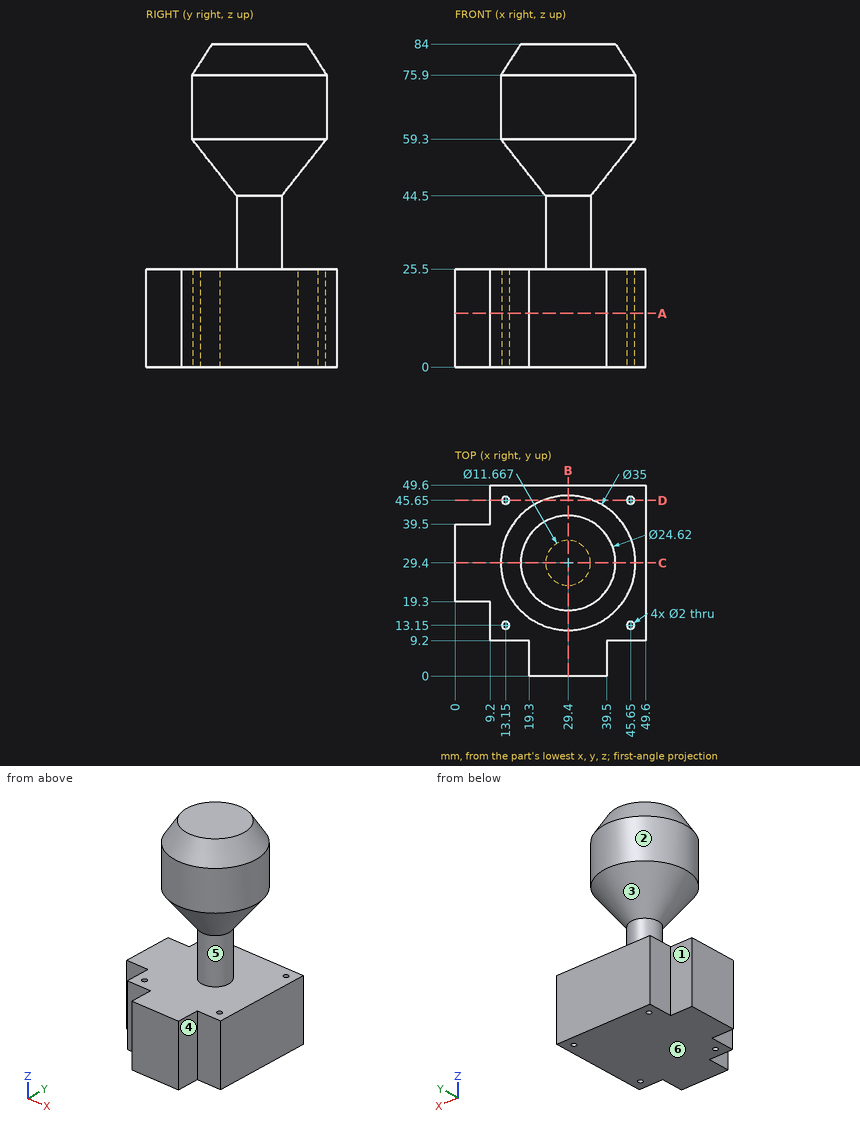
Could you check a few things on this drawing? It's one solid part, dimensions in mm from its lowest x, y, z. A direction names the side the tool comes from. Coordinates: 2 decimals unless noted, no trailing zeros. Write each loop counter-clockwise with the first axis right and the second up, starting at its lowest first coordinate (ties: lowest second). Pieces come first, ordered by that corner, then holes. Notation, with made-up numbers: M -23.75,-30.5 L -0.75,-30.5 A25 cw -0.75,-9.5 Z; hole C -38,28 d3. An arc over 180 degrees is marked long. Answer as CSV lines item,"result". Start each with the question number.
Q1. Suppose I cut it at D-D, the plane y = 45.65. State how many separate pieces and enclosed holes the cut face has, then the cut area to 3 significant figures.
Q2. If we mould it in two halves opening along Z, with no side actions, what happens to the marked faces 4, 5 and 6? For each: pulls with the +Z half, pulls with the -Z half, needs draft (parallel to the pull), parting line crosses it, or undercut.
Q3. Will these pins go through, and if not, where does the flat tip stop? pin 1 Ø11 at (y, z) = (13, 6.5) entering from -X; pin 2 Ø2.5 at (x, y) = (45.65, 45.65) entering from -Z; pin 3 Ø3 at (x, z) = (14, 14.5) entering from -Y; pin 4 Ø4 at (x, y) = (43, 40.5) entering from +Z (1 decimal).
Q4. Suppose I cut it at A-A, the plane z = 14. List the corners of the cut face in (x, y) for me, then the cut area to 3 significant figures.
Q5. I need wall thicknesses on probe 1 along Y at (x, z) = (45.65, 19); probe 2 along Z at (x, y) = (2, 27). Which ranges of each line are inside material? Lowest first, please. Write a range as [from, to].
Q6. Suppose I cut it at B-B, the plane x = 29.4. List the corners of the cut face in (y, z) for me.
Q7. For the marked faces 1, 2 and 3, which set-ups out of +Z, -Z, +X, -X, +Y, -Y let a thin tool reach every point of the face, with its end or its side?
Entries:
1,separate pieces,"4"
1,enclosed holes,"0"
1,area,"1,170 mm²"
2,face 4,"needs draft"
2,face 5,"undercut"
2,face 6,"pulls with the -Z half"
3,pin 1,"stops at x = 9.2"
3,pin 2,"stops at z = 0"
3,pin 3,"stops at y = 9.2"
3,pin 4,"stops at z = 78.9"
4,outline,"M 0,19.3 L 9.2,19.3 L 9.2,9.2 L 19.3,9.2 L 19.3,0 L 39.5,0 L 39.5,9.2 L 49.6,9.2 L 49.6,49.6 L 9.2,49.6 L 9.2,39.5 L 0,39.5 Z; hole C 13.15,13.15 d2; hole C 13.15,45.65 d2; hole C 45.65,13.15 d2; hole C 45.65,45.65 d2"
4,area,"1,990 mm²"
5,probe 1,"y = [9.2, 12.15], [14.15, 44.65], [46.65, 49.6]"
5,probe 2,"z = [0, 25.5]"
6,outline,"M 0,0 L 49.6,0 L 49.6,25.5 L 35.23,25.5 L 35.23,44.5 L 46.9,59.3 L 46.9,75.9 L 41.71,84 L 17.09,84 L 11.9,75.9 L 11.9,59.3 L 23.57,44.5 L 23.57,25.5 L 0,25.5 Z"
7,face 1,"+Z, -Z, -X, +Y"
7,face 2,"+Z"
7,face 3,"none"
